Work out the finished part from the listing and answer in its coordinate system (mm). A direction names the side the tool comes from. Give positions to 0.01 mm unless a question says otherwise; leave off trailing zeros. Order: outer loops, then holes, each group sorted by start corner. A loop starts at its lowest first (then second) coordinate and runs counter-clockwise, first axis right, second up. Notation, with made-up numbers: M 20.25,-16.75 L 67.25,-16.75 A16 ccw 67.25,11.25 Z; hole C 59,19 d10. An arc over 180 degrees is marked long. One line per item, written item: value.
from build123d import *

# Parameters (mm, degrees)
SKETCH1_W           = 70
SKETCH1_H           = 100
BOSS_EXTRUDE1_DEPTH = 10
SKETCH2_R           = 2.5
CUT_EXTRUDE1_DEPTH  = 11
SKETCH3_R           = 1.5
CUT_EXTRUDE2_DEPTH  = 11
SKETCH4_R           = 3.45
CUT_EXTRUDE3_DEPTH  = 4
SKETCH5_R           = 2
CUT_EXTRUDE4_DEPTH  = 11


with BuildPart() as part:
    # Sketch1 → Boss-Extrude1 (new body)
    with BuildSketch(Plane.XY):
        Rectangle(SKETCH1_W, SKETCH1_H)
    extrude(amount=BOSS_EXTRUDE1_DEPTH)

    # Sketch2 → Cut-Extrude1 (cut, through all)
    with BuildSketch(Plane(origin=(0, 0, 0), x_dir=(-1, 0, 0), z_dir=(0, 0, -1))):
        with Locations((-25, 45)):
            Circle(SKETCH2_R)
        with Locations((25, 45)):
            Circle(SKETCH2_R)
        with Locations((-25, -45)):
            Circle(SKETCH2_R)
        with Locations((25, -45)):
            Circle(SKETCH2_R)
    extrude(amount=-CUT_EXTRUDE1_DEPTH, mode=Mode.SUBTRACT)

    # Sketch3 → Cut-Extrude2 (cut, through all)
    with BuildSketch(Plane(origin=(0, 0, 0), x_dir=(-1, 0, 0), z_dir=(0, 0, -1))):
        with Locations((9, 21)):
            Circle(SKETCH3_R)
        with Locations((9, 45)):
            Circle(SKETCH3_R)
        with Locations((-9, 21)):
            Circle(SKETCH3_R)
        with Locations((-9, 45)):
            Circle(SKETCH3_R)
        with Locations((9, -45)):
            Circle(SKETCH3_R)
        with Locations((9, -21)):
            Circle(SKETCH3_R)
        with Locations((-9, -45)):
            Circle(SKETCH3_R)
        with Locations((-9, -21)):
            Circle(SKETCH3_R)
    extrude(amount=-CUT_EXTRUDE2_DEPTH, mode=Mode.SUBTRACT)

    # Sketch4 → Cut-Extrude3 (cut)
    with BuildSketch(Plane.XY.offset(10)):
        with Locations((-9, 45)):
            Circle(SKETCH4_R)
        with Locations((-9, 21)):
            Circle(SKETCH4_R)
        with Locations((9, 21)):
            Circle(SKETCH4_R)
        with Locations((9, 45)):
            Circle(SKETCH4_R)
        with Locations((9, -21)):
            Circle(SKETCH4_R)
        with Locations((-9, -21)):
            Circle(SKETCH4_R)
        with Locations((-9, -45)):
            Circle(SKETCH4_R)
        with Locations((9, -45)):
            Circle(SKETCH4_R)
    extrude(amount=-CUT_EXTRUDE3_DEPTH, mode=Mode.SUBTRACT)

    # Sketch5 → Cut-Extrude4 (cut, through all)
    with BuildSketch(Plane.XY.offset(10)):
        with Locations((0, -11)):
            Circle(SKETCH5_R)
        with Locations((0, 11)):
            Circle(SKETCH5_R)
    extrude(amount=-CUT_EXTRUDE4_DEPTH, mode=Mode.SUBTRACT)


solid = part.part
(1) Which of the six approach directions +Z, -Z, +X, -X, +Y, -Y give full straight-line access (tool end or side, diameter ignored) to faces 4 (the cylindrical face through (9.325, 43.536, 2.958)), 5 (the flat face through (-8.3, 19.5, 6))?
Findings:
face 4: +Z, -Z
face 5: +Z
(2) Section A-A, the plane x = 25 is taken. Give the vertices of the cut face in (y, z).
Findings:
outline: M -50,0 L -47.5,0 L -47.5,10 L -50,10 Z; M -42.5,0 L 42.5,0 L 42.5,10 L -42.5,10 Z; M 47.5,0 L 50,0 L 50,10 L 47.5,10 Z
(3) Section C-C, the plane z = 2.5 is taken. Give the number of separate pieces and of enclosed holes in the cut face, then the cut area to 3 significant figures.
Findings:
separate pieces: 1
enclosed holes: 14
area: 6,840 mm^2
(4) Given P1, Ø4, axis at x = 9, y = 21, coming from the +Z side, flat-ended and moving along its own axis, determine where the tip first touches the part or whether it passes through.
Findings:
P1: stops at z = 6
(5) Find the intervals of material crossed by probe 1 along Y at (x, z) = (-9, 1.55); probe 2 along Y at (x, z) = (9, 8.85); probe 3 along Y at (x, z) = (27, 5), in increasing order. Write a range as from..to.
Findings:
probe 1: y = -50..-46.5, -43.5..-22.5, -19.5..19.5, 22.5..43.5, 46.5..50
probe 2: y = -50..-48.45, -41.55..-24.45, -17.55..17.55, 24.45..41.55, 48.45..50
probe 3: y = -50..-46.5, -43.5..43.5, 46.5..50
(6) Determine the mould class of faces 1 (the flat face through (0, -50, 5)), 2 (the flat face through (35, -1, 5)), 3 (the cylindrical face through (8.252, -48.368, 8.028)) for opening direction X: pulls with the +X half, pulls with the -X half, needs draft (parallel to the pull), parting line crosses it, or undercut.
Findings:
face 1: needs draft
face 2: pulls with the +X half
face 3: undercut
(7) Section B-B, the plane y = 11 is taken. Give the vertices of the cut face in (x, z).
Findings:
outline: M -35,0 L -2,0 L -2,10 L -35,10 Z; M 2,0 L 35,0 L 35,10 L 2,10 Z
(8) Section D-D, the plane y = -45 is taken. Give the vertices of the cut face in (x, z).
Findings:
outline: M -35,0 L -27.5,0 L -27.5,10 L -35,10 Z; M -22.5,0 L -10.5,0 L -10.5,6 L -12.45,6 L -12.45,10 L -22.5,10 Z; M -7.5,0 L 7.5,0 L 7.5,6 L 5.55,6 L 5.55,10 L -5.55,10 L -5.55,6 L -7.5,6 Z; M 10.5,0 L 22.5,0 L 22.5,10 L 12.45,10 L 12.45,6 L 10.5,6 Z; M 27.5,0 L 35,0 L 35,10 L 27.5,10 Z
